For this review, take the finished solid that the model builds, in its own axes (mm). A direction names the side the tool comes from. Give positions to 0.01 mm unless a question says otherwise; leave off trailing zeros. Order: outer loops, then holes, each group sorted by start corner. A loop starts at its lowest first (then second) coordinate and runs counter-clockwise, first axis right, second up.
from build123d import *

# Parameters (mm, degrees)
BOSS_EXTRUDE1_DEPTH = 25
SKETCH3_R           = 2.1
CUT_EXTRUDE1_DEPTH  = 107.086049978
SKETCH3_3_R         = 4
SKETCH3_3_R_2       = 2.1
CUT_EXTRUDE2_DEPTH  = 5
FILLET1_R           = 2
CHAMFER1_SIZE       = 1


with BuildPart() as part:
    # Sketch2 → Boss-Extrude1 (new body)
    with BuildSketch(Plane.XY):
        Polygon((0, 0), (87, 0), (87, 38.5), (83, 38.5), (83, 40.5), (93, 44.5), (93, 38.5), (93, -10), (87, -10), (0, -10), (-6, -10), (-6, 38.5), (-6, 44.5), (4, 40.5), (4, 38.5), (0, 38.5), align=None)
    extrude(amount=BOSS_EXTRUDE1_DEPTH)

    # Sketch3 → Cut-Extrude1 (cut, through all)
    with BuildSketch(Plane(origin=(0, 0, 0), x_dir=(1, 0, 0), z_dir=(0, 1, 0))):
        with Locations(Location((16, -12.5, 0), (0, 0, 180))):
            Circle(SKETCH3_R)
        with Locations(Location((71, -12.5, 0), (0, 0, 180))):
            Circle(SKETCH3_R)
    extrude(amount=-CUT_EXTRUDE1_DEPTH, mode=Mode.SUBTRACT)

    # Sketch3_3 → Cut-Extrude2 (cut)
    # profile 1 of 2: a face of its own
    with BuildSketch(Plane(origin=(0, 0, 0), x_dir=(1, 0, 0), z_dir=(0, 1, 0))):
        with Locations(Location((16, -12.5, 0), (0, 0, 180))):
            Circle(SKETCH3_3_R)
        with Locations(Location((16, -12.5, 0), (0, 0, 180))):
            Circle(SKETCH3_3_R_2, mode=Mode.SUBTRACT)
    # profile 2 of 2: a face of its own
    with BuildSketch(Plane(origin=(0, 0, 0), x_dir=(1, 0, 0), z_dir=(0, 1, 0))):
        with Locations(Location((71, -12.5, 0), (0, 0, 180))):
            Circle(SKETCH3_3_R)
        with Locations(Location((71, -12.5, 0), (0, 0, 180))):
            Circle(SKETCH3_3_R_2, mode=Mode.SUBTRACT)
    extrude(amount=-CUT_EXTRUDE2_DEPTH, mode=Mode.SUBTRACT)

    # Fillet1
    fillet1_edges = [part.edges().sort_by_distance(p)[0] for p in [
        (83, 40.5, 12.5),
        (93, 44.5, 12.5),
        (-6, 44.5, 12.5),
        (4, 40.5, 12.5),
    ]]
    fillet(fillet1_edges, radius=FILLET1_R)

    # Chamfer1
    chamfer1_edges = [part.edges().sort_by_distance(p)[0] for p in [
        (2, 38.5, 25),
        (0, 19.25, 25),
        (85, 38.5, 25),
        (87, 19.25, 25),
        (43.5, 0, 25),
        (85, 38.5, 0),
        (87, 19.25, 0),
        (43.5, 0, 0),
        (2, 38.5, 0),
        (0, 19.25, 0),
        (93, -10, 12.5),
        (43.5, -10, 0),
        (-6, -10, 12.5),
        (43.5, -10, 25),
    ]]
    chamfer(chamfer1_edges, length=CHAMFER1_SIZE)


solid = part.part
1) We need section B-B on y = 33.5. Give the boundary of the cut face in (x, z), then the cut area to 3 significant figures.
Answer sheet:
outline: (-6, 0) - (-1, 0) - (0, 1) - (0, 24) - (-1, 25) - (-6, 25) - close; (87, 1) - (88, 0) - (93, 0) - (93, 25) - (88, 25) - (87, 24) - close
area: 298 mm2
2) We need section A-A on x = 16. Give the boundary of the cut face in (y, z).
Answer sheet:
outline: (-10, 1) - (-9, 0) - (-1, 0) - (0, 1) - (0, 8.5) - (-5, 8.5) - (-5, 10.4) - (-10, 10.4) - close; (-10, 14.6) - (-5, 14.6) - (-5, 16.5) - (0, 16.5) - (0, 24) - (-1, 25) - (-9, 25) - (-10, 24) - close
3) Tool access review of faces 1 (the face through (67.185, -2.465, 13.701)), 2 (the face through (-0.3, 42.22, 12.32)), 3 (the face through (-6, 17, 12)), 4 (the face through (0, 20, 12)): name each direction out of +Z, -Z, +X, -X, +Y, -Y from which nothing blocks a thin tool from reaching the whole face with its end or side.
Answer sheet:
face 1: +Y
face 2: +Z, -Z, +Y
face 3: +Z, -Z, -X, +Y, -Y
face 4: +Z, -Z
4) To check wall thickness, follow line 1 (X direction, y = 9.5, z = 3); line 2 (Z direction, x = 16, y = -1.3); line 3 (Z direction, x = 71, y = -6). State the ranges of each line that lie inside material, in increasing order.
Answer sheet:
line 1: x = -6 to 0, 87 to 93
line 2: z = 0 to 8.5, 16.5 to 25
line 3: z = 0 to 10.4, 14.6 to 25
5) Clearance check with flat-ended pins moving along their axes: pin 1 (5.5 mm diameter, centred on x = 16, z = 12.5, fed in from +Y); pin 2 (1 mm diameter, centred on x = 8, z = 10, fed in from +Y). State where each tip first meets the part, or that it passes through.
Answer sheet:
pin 1: stops at y = -5
pin 2: stops at y = 0
6) Draft analysis for pull direction Y (two halves, no side actions). For faces 5 (the face through (87, 19, 12)), 6 (the face through (18.95, -2.46, 15.2)), 7 (the face through (69, -5, 11)), state which applies: +Y half, -Y half, draft (parallel to the pull), parting line (faces both ways), or undercut.
Answer sheet:
face 5: undercut
face 6: draft
face 7: +Y half
7) We need section C-C on z = 12.5. Count the separate pieces of the cut face and the enclosed holes in it, then the cut area to 3 significant figures.
Answer sheet:
separate pieces: 3
enclosed holes: 0
area: 1,400 mm2
8) We need section D-D on z = 19.5. Give the boundary of the cut face in (x, y), then the cut area to 3 significant figures.
Answer sheet:
outline: (-6, -9) - (-5, -10) - (92, -10) - (93, -9) - (93, 41.55) arc R2 ccw to (90.26, 43.4) - (84.26, 41) arc R2 ccw to (83, 39.15) - (83, 38.5) - (87, 38.5) - (87, 0) - (0, 0) - (0, 38.5) - (4, 38.5) - (4, 39.15) arc R2 ccw to (2.74, 41) - (-3.26, 43.4) arc R2 ccw to (-6, 41.55) - close
area: 1,530 mm2
